from build123d import *

# Parameters (mm, degrees)
SKETCH_1_R          = 6.75
EXTRUDE_1_DEPTH     = 2.5
SKETCH_2_R          = 3.05
CUT_EXTRUDE_1_DEPTH = 3.5
SKETCH_3_R          = 5.75
CUT_EXTRUDE_2_DEPTH = 1


with BuildPart() as part:
    # 草图1 → 凸台-拉伸1 (new body)
    with BuildSketch(Plane.XY):
        Circle(SKETCH_1_R)
    extrude(amount=EXTRUDE_1_DEPTH)

    # 草图2 → 切除-拉伸1 (cut, through all)
    with BuildSketch(Plane.XY.offset(2.5)):
        Circle(SKETCH_2_R)
    extrude(amount=-CUT_EXTRUDE_1_DEPTH, mode=Mode.SUBTRACT)

    # 草图3 → 切除-拉伸2 (cut)
    with BuildSketch(Plane.XY.offset(2.5)):
        Circle(SKETCH_3_R)
    extrude(amount=-CUT_EXTRUDE_2_DEPTH, mode=Mode.SUBTRACT)


solid = part.part
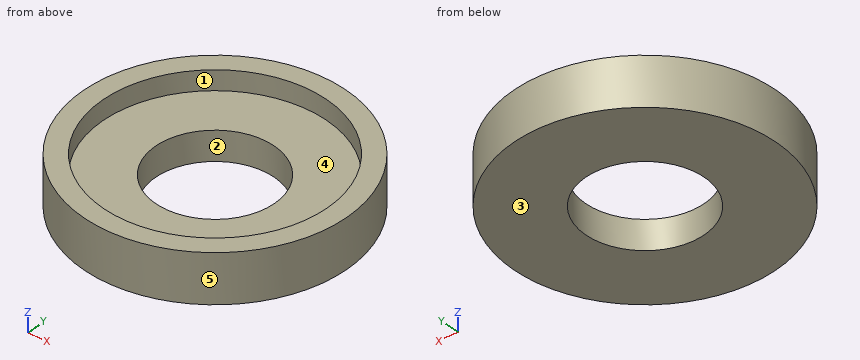
Source: CAD feature listing. Evaluate the final solid. Frame: model axes, mm. Face numbers are marked on the shaded views. A direction names the side the tool comes from. Round coordinates to 2 decimals unless told otherwise and drop trailing zeros. Order: outer loops, then holes, each group sorted by start corner. A loop starts at its lowest first (then second) coordinate and runs counter-clockwise, first axis right, second up. Notation, with made-up numbers: (-2, 88) -> (55, 88) arc R13 ccw to (55, 106) -> close; hole circle Ø8 at (-25.5, 33). An arc over 180 degrees is marked (long way). Answer as CSV lines item,"result".
Item 1: Section A-A, the plane y = 0. Return loops of the section in (x, z), plus the area to 3 significant figures.
A:
outline,"(-6.75, 0) -> (-3.05, 0) -> (-3.05, 1.5) -> (-5.75, 1.5) -> (-5.75, 2.5) -> (-6.75, 2.5) -> close; (3.05, 0) -> (6.75, 0) -> (6.75, 2.5) -> (5.75, 2.5) -> (5.75, 1.5) -> (3.05, 1.5) -> close"
area,"13.1 mm²"
Item 2: Pull-direction query (X, two-part tool) for the marked faces 3, 4 and 5; classes: pulls with the +X half, pulls with the -X half, needs draft (parallel to the pull), parting line crosses it, or undercut.
A:
face 3,"needs draft"
face 4,"undercut"
face 5,"parting line crosses it"
Item 3: Section D-D, the plane y = 5.5. Return loops of the section in (x, z), plus the area to 3 significant figures.
A:
outline,"(-3.91, 0) -> (3.91, 0) -> (3.91, 2.5) -> (1.68, 2.5) -> (1.68, 1.5) -> (-1.68, 1.5) -> (-1.68, 2.5) -> (-3.91, 2.5) -> close"
area,"16.2 mm²"
Item 4: Section C-C, the plane z = 2.2. Return loops of the section in (x, y), plus the area to 3 significant figures.
A:
outline,"circle Ø13.5 at (0, 0); hole circle Ø11.5 at (0, 0)"
area,"39.3 mm²"
Item 5: Reachability of the marked faces 1 and 2 from +Z, -Z, +X, -X, +Y, -Y: full face, straight path, thin tool, end or side. Return the list, or none.
A:
face 1,"+Z"
face 2,"+Z, -Z"
Item 6: Line query: L1, parallel to Y at x = 0, z = 2.15; L2, parallel to Y at x = 0, z = 0.8; L3, parallel to Z at x = 1.25, y = 5.25. Output: solid intervals per line, ascending.
A:
L1,"-6.75 to -5.75, 5.75 to 6.75"
L2,"-6.75 to -3.05, 3.05 to 6.75"
L3,"0 to 1.5"
Item 7: Pin query (flat end, axial travel): pin 1 Ø1 at (x, z) = (1, 1.5) entering from -Y; pin 2 Ø1.5 at (x, y) = (2, -1.5) entering from +Z. Return the tip coordinate at first contact, or that it passes through.
A:
pin 1,"y = -6.73"
pin 2,"z = 1.5"
